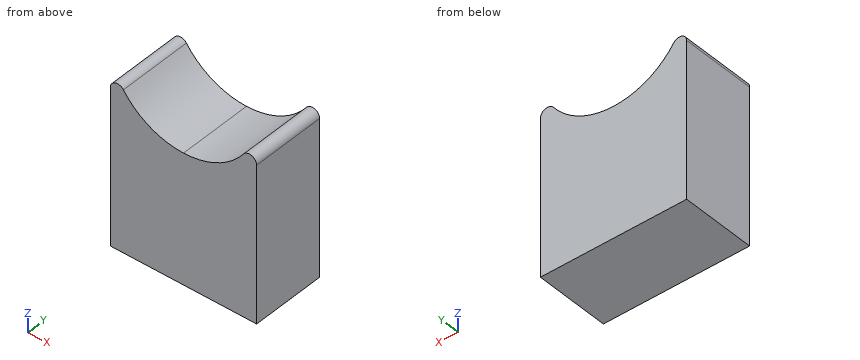
```python
from build123d import *

# Parameters (mm, degrees)
SKETCH1_W           = 6.1
SKETCH1_H           = 5.4
BOSS_EXTRUDE2_DEPTH = 3.1
FILLET1_R           = 0.3


with BuildPart() as part:
    # Sketch1 → Boss-Extrude2 (new body)
    with BuildSketch(Plane(origin=(0, 0, 0), x_dir=(1, 0, 0), z_dir=(0, 1, 0))):
        Rectangle(SKETCH1_W, SKETCH1_H)
        with BuildLine():
            Line((0, -2.7), (-3.05, -2.7))
            Line((-3.05, -2.7), (-3.05, -5.245473175))
            ThreePointArc((-3.05, -5.245473175), (-1.986324098, -3.419975509), (0, -2.7))
        make_face()
        with BuildLine():
            Line((3.05, -2.7), (0, -2.7))
            ThreePointArc((0, -2.7), (1.986324098, -3.419975509), (3.05, -5.245473175))
            Line((3.05, -5.245473175), (3.05, -2.7))
        make_face()
    extrude(amount=BOSS_EXTRUDE2_DEPTH)

    # Fillet1
    fillet1_edges = [part.edges().sort_by_distance(p)[0] for p in [
        (3.05, 1.55, 5.245473175),
        (-3.05, 1.55, 5.245473175),
    ]]
    fillet(fillet1_edges, radius=FILLET1_R)


solid = part.part
```
Work out the finished part from the listing and answer in its coordinate system (mm). Give positions to 0.01 mm unless a question says otherwise; leave off trailing zeros. Loops run counter-clockwise (first coordinate to the right, second up) from the corner with the lowest first, then second, coordinate; pieces in that order, holes last. Notation, with made-up numbers: (-11, 25) - (26, 25) arc R12 cw to (26, 47) - close; hole circle Ø4 at (-10.5, 27). An arc over 180 degrees is marked (long way). One line per question, with ' | ' between items.
(1) The part is cut by section A-A (y = 1.55). Write down the section's boundary in (x, z).
Recorded:
outline: (-3.05, -2.7) - (3.05, -2.7) - (3.05, 3.8) arc R0.3 ccw to (2.51, 3.98) arc R3.1 cw to (-2.51, 3.98) arc R0.3 ccw to (-3.05, 3.8) - close
(2) The part is cut by section B-B (x = -1). Write down the section's boundary in (y, z).
Recorded:
outline: (0, -2.7) - (3.1, -2.7) - (3.1, 2.87) - (0, 2.87) - close
(3) Straight lines are drawn through the part: probe 1 along X at (y, z) = (2.8, 3.5); probe 2 along Z at (x, y) = (0.5, 2.45); probe 3 along Z at (x, y) = (-1.25, 0.3). For each, find the intervals that lie inside material, in ascending order.
Recorded:
probe 1: x = -3.05 to -2.08, 2.08 to 3.05 | probe 2: z = -2.7 to 2.74 | probe 3: z = -2.7 to 2.96
(4) The part is cut by section C-C (x = 1.25). Write down the section's boundary in (y, z), then the cut area to 3 significant figures.
Recorded:
outline: (0, -2.7) - (3.1, -2.7) - (3.1, 2.96) - (0, 2.96) - close | area: 17.6 mm²
